Autodesk Inventor part; units mm, degrees
ref_plane "Work Plane1" through (-12, 0, 0) normal (0, 0, 1) x (1, 0, 0)
ref_plane "YZ Plane" through (0, 0, 0) normal (1, 0, 0) x (0, 1, 0)
ref_plane "XZ Plane" through (0, 0, 0) normal (0, 1, 0) x (-1, 0, 0)
sketch "Sketch1" plane through (0, 0, 0) normal (0, 1, 0) x (-1, 0, 0)
  line L0 (12, 40) -> (-12, 40)
  line L1 (-12, 40) -> (-12, -40)
  line L2 (-12, -40) -> (12, -40)
  line L3 (12, -40) -> (12, 40)
  line L4 (12, 40) -> (-12, -40) construction
  line L5 (-12, 40) -> (12, -40) construction
  point P0 (0, 0)
  dimension "d0" = 24
  dimension "d1" = 80
extrude "Extrusion1" add sketch "Sketch1" along normal blind 32.5
sketch "Sketch2" plane through (12, 0, 40) normal (1, 0, 0) x (0, 0, -1)
  circle A0 centre (40, 16.25) radius 3
  line L0 (0, 0) -> (0, 32.5)
  line L1 (0, 32.5) -> (80, 32.5)
  point P0 (40, 0)
  point P1 (40, 32.5)
  dimension "d4" = 6
  dimension "d5" = 40
  dimension "d6" = 16.25
extrude "Extrusion2" cut sketch "Sketch2" against normal blind 5
ref_plane "Work Plane1" through (-12, 0, 0) normal (0, 0, 1) x (1, 0, 0)
sketch "Sketch5" plane through (-12, 0, 0) normal (0, 0, 1) x (1, 0, 0)
  circle A0 centre (-4, 16.25) radius 2
  line L0 (0, 0) -> (0, 32.5)
  line L1 (24, 32.5) -> (0, 32.5)
  arc A1 (-4, 20.25) -> (-4, 12.25) centre (-4, 16.25) ccw
  line L2 (-4, 12.25) -> (0, 12.25)
  line L3 (-4, 20.25) -> (0, 20.25)
  point P0 (12, 0)
  dimension "d9" = 4
  dimension "d10" = 4
  dimension "d11" = 16.25
  dimension "d12" = 4
extrude "Extrusion3" add sketch "Sketch5" along normal blind 7.5 and the other way blind 7.5
sketch "Sketch7" plane through (-12, 0, -7.5) normal (0, 0, -1) x (-1, 0, 0)
  line L0 (0, 12.25) -> (4, 12.25)
  arc A0 (4, 12.25) -> (4, 20.25) centre (4, 16.25) ccw
  line L1 (4, 20.25) -> (0, 20.25)
  line L2 (0, 12.25) -> (0, 20.25)
  circle A1 centre (4, 16.25) radius 2
  line L3 (4, 14.25) -> (7.4641, 14.25)
  line L4 (4, 18.25) -> (7.4641, 18.25)
  point P0 (-12, 0)
extrude "Extrusion4" cut sketch "Sketch7" against normal blind 2 contours L3 A1 L4 A0
mirror "Mirror1" about plane through (-12, 0, 0) normal (0, 0, 1) of "Extrusion4"
fillet "Fillet2" radius 5 4 edges at (-12, 16.25, 40) (-12, 16.25, -40) (12, 16.25, -40) (12, 16.25, 40)
properties part number "Camera"
The listing builds one solid part. Answer for the finished solid, in the listing's coordinates (mm). A direction names the side the tool comes from. Round coordinates to 2 decimals unless told otherwise and drop trailing zeros. Order: outer loops, then holes, each group sorted by start corner. A loop starts at its lowest first (then second) coordinate and runs counter-clockwise, first axis right, second up. Notation, with made-up numbers: (82.5, 18) -> (123.5, 18) arc R28 ccw to (123.5, 42) -> close; hole circle Ø11 at (-1, 32.25). An arc over 180 degrees is marked (long way). One line per item, written item: value.
Item 1: Find section A-A, the plane z = 0. Give the vertices of the cut face in (x, y).
Taken from the geometry:
outline: (-16, 12.25) -> (-12, 12.25) -> (-12, 0) -> (12, 0) -> (12, 13.25) -> (7, 13.25) -> (7, 19.25) -> (12, 19.25) -> (12, 32.5) -> (-12, 32.5) -> (-12, 20.25) -> (-16, 20.25) arc R4 ccw to start; hole circle Ø4 at (-16, 16.25)
Item 2: Given P1, Ø1, axis at x = -17.5, z = -7, coming from the -Y side; P2, Ø4.5, axis at x = -18, y = 15.5, coming from the +Z side; P3, Ø3, axis at x = -19, y = 17, coming from the -Z side, each flat-ended and moving along its own axis, determine where each tip first touches the part or whether it passes through.
Taken from the geometry:
P1: stops at y = 12.38
P2: stops at z = 7.5
P3: stops at z = -7.5
Item 3: Find section C-C, the plane x = -17. Give the vertices of the cut face in (y, z).
Taken from the geometry:
outline: (12.38, -7.5) -> (14.25, -7.5) -> (14.25, -5.5) -> (14.52, -5.5) -> (14.52, 5.5) -> (14.25, 5.5) -> (14.25, 7.5) -> (12.38, 7.5) -> close; (17.98, -5.5) -> (18.25, -5.5) -> (18.25, -7.5) -> (20.12, -7.5) -> (20.12, 7.5) -> (18.25, 7.5) -> (18.25, 5.5) -> (17.98, 5.5) -> close
Item 4: Find section D-D, the plane y = 30.5. Give the vertices of the cut face in (x, z).
Taken from the geometry:
outline: (-12, -35) arc R5 ccw to (-7, -40) -> (7, -40) arc R5 ccw to (12, -35) -> (12, 35) arc R5 ccw to (7, 40) -> (-7, 40) arc R5 ccw to (-12, 35) -> close
Item 5: For a pull along Z with two mould halves and no side action, classify faces 1 (the flat face through (-14, 15, 7.5)), 2 (the flat face through (-14, 12.25, 0)), 3 (the cylindrical face through (9.54, 13.32, 0.65)) as released by +Z, released by -Z, zero draft, split by the parting line, or undercut.
Taken from the geometry:
face 1: released by +Z
face 2: zero draft
face 3: undercut
Item 6: Find section B-B, the plane y = 16.25. Give the vertices of the cut face in (x, z).
Taken from the geometry:
outline: (-20, -5.5) -> (-18, -5.5) -> (-18, 5.5) -> (-20, 5.5) -> close; (-14, -7.5) -> (-12, -7.5) -> (-12, -35) arc R5 ccw to (-7, -40) -> (7, -40) arc R5 ccw to (12, -35) -> (12, -3) -> (7, -3) -> (7, 3) -> (12, 3) -> (12, 35) arc R5 ccw to (7, 40) -> (-7, 40) arc R5 ccw to (-12, 35) -> (-12, 7.5) -> (-14, 7.5) -> close
Item 7: Straight lines are drawn through the part: L1, parallel to X at y = 16, z = 2; L2, parallel to Y at x = -16, z = -4; L3, parallel to X at y = 16.25, z = -3.25. For each, find the intervals that lie inside material, in ascending order.
Taken from the geometry:
L1: x = -19.99 to -17.98, -14.02 to 7
L2: y = 12.25 to 14.25, 18.25 to 20.25
L3: x = -20 to -18, -14 to 12
Item 8: For faces 4 (the flat face through (-14, 15, -7.5)), 5 (the cylindrical face through (10, 16, 39)), 6 (the flat face through (-18.5, 16.3, 5.5)), 7 (the flat face through (7, 16, 0)), determine the directions among +Z, -Z, +X, -X, +Y, -Y from which every point of the face is accessible in a straight line to the end or side of a thin tool.
Taken from the geometry:
face 4: -Z, -X, +Y, -Y
face 5: +Z, +X, +Y, -Y
face 6: +Z, -X
face 7: +X
